Source: CAD feature listing. Evaluate the final solid. Frame: model axes, mm. A direction names the side the tool comes from. Give positions to 0.01 mm unless a question says otherwise; leave off trailing zeros. Write each loop counter-clockwise with the first axis right and the second up, starting at its lowest first coordinate (ties: lowest second). Pieces come first, ordered by that corner, then holes. Notation, with made-up numbers: (-8, 5) -> (4, 5) arc R27 cw to (4, 43) -> close; hole circle Ø1 at (72, 82). An arc over 180 degrees is marked (long way). Write item = value, one per line.
from build123d import *

# Parameters (mm, degrees)
SKETCH1_R            = 18.25
BOSS_EXTRUDE1_DEPTH  = 44.5
BOSS_EXTRUDE2_DEPTH  = 32
SKETCH3_R            = 4.75
CUT_EXTRUDE2_DEPTH   = 32
CUT_EXTRUDE3_DEPTH   = 32
SKETCH5_R            = 14.25
CUT_EXTRUDE4_DEPTH   = 4
CHAMFER1_SIZE        = 0.5
FILLET1_R            = 0.75
SKETCH6_R            = 12
CUT_EXTRUDE5_DEPTH   = 3
SKETCH7_R            = 13
BOSS_EXTRUDE3_DEPTH  = 5.5
FILLET2_R            = 1.8
SKETCH8_R            = 15.875
BOSS_EXTRUDE4_DEPTH  = 3.75
SKETCH9_R            = 14.5
BOSS_EXTRUDE5_DEPTH  = 4.75
SKETCH10_R           = 15.875
BOSS_EXTRUDE6_DEPTH  = 3.75
FILLET3_R            = 1
FILLET3_OF_MIRROR1_R = 1
SKETCH11_R           = 12.75
CUT_EXTRUDE6_DEPTH   = 79.75
SKETCH12_R           = 8
CUT_EXTRUDE7_DEPTH   = 32.75


with BuildPart() as part:
    # Sketch1 → Boss-Extrude1 (new body)
    with BuildSketch(Plane(origin=(0, 0, 0), x_dir=(1, 0, 0), z_dir=(0, 1, 0))):
        with Locations(Location((0, 0, 0), (0, 0, 270))):
            Circle(SKETCH1_R)
    extrude(amount=BOSS_EXTRUDE1_DEPTH)

    # Sketch2 → Boss-Extrude2 (add)
    with BuildSketch(Plane.XZ):
        with BuildLine():
            Line((25.5, 0), (25.5, -43))
            Line((25.5, -43), (-25.5, -43))
            Line((-25.5, -43), (-25.5, 0))
            ThreePointArc((-25.5, 0), (-20.032746784, 3.769396236), (-15.896474532, 8.964630358))
            ThreePointArc((-15.896474532, 8.964630358), (0, -18.25), (15.896474532, 8.964630358))
            ThreePointArc((15.896474532, 8.964630358), (20.032746784, 3.769396236), (25.5, 0))
        make_face()
    extrude(amount=-BOSS_EXTRUDE2_DEPTH)

    # Sketch3 → Cut-Extrude2 (cut)
    with BuildSketch(Plane(origin=(0, 32, 0), x_dir=(1, 0, 0), z_dir=(0, 1, 0))):
        with Locations(Location((-16.5, 34.25, 0), (0, 0, 270))):
            Circle(SKETCH3_R)
        with Locations(Location((16.5, 34.25, 0), (0, 0, 90))):
            Circle(SKETCH3_R)
    extrude(amount=-CUT_EXTRUDE2_DEPTH, mode=Mode.SUBTRACT)

    # Sketch4 → Cut-Extrude3 (cut)
    with BuildSketch(Plane(origin=(0, 32, 0), x_dir=(1, 0, 0), z_dir=(0, 1, 0))):
        with BuildLine():
            Line((16.25, 43), (-16.25, 43))
            ThreePointArc((-16.25, 43), (-11.008714433, 41.194952561), (-7.860592425, 36.632212324))
            ThreePointArc((-7.860592425, 36.632212324), (-5.818294481, 32.970747376), (-2.07874831, 31.075199726))
            ThreePointArc((-2.07874831, 31.075199726), (-1.040129155, 31.016729364), (0, 31))
            ThreePointArc((0, 31), (1.040129155, 31.016729364), (2.07874831, 31.075199726))
            ThreePointArc((2.07874831, 31.075199726), (5.818294481, 32.970747376), (7.860592425, 36.632212324))
            ThreePointArc((7.860592425, 36.632212324), (11.008714433, 41.194952561), (16.25, 43))
        make_face()
        with BuildLine():
            Line((-16.75, 43), (-25.5, 43))
            Line((-25.5, 43), (-25.5, 34.25))
            ThreePointArc((-25.5, 34.25), (-22.901195105, 40.401195105), (-16.75, 43))
        make_face()
        with BuildLine():
            Line((25.5, 43), (16.75, 43))
            ThreePointArc((16.75, 43), (22.901195105, 40.401195105), (25.5, 34.25))
            Line((25.5, 34.25), (25.5, 43))
        make_face()
    extrude(amount=-CUT_EXTRUDE3_DEPTH, mode=Mode.SUBTRACT)

    # Sketch5 → Cut-Extrude4 (cut)
    with BuildSketch(Plane(origin=(0, 44.5, 0), x_dir=(1, 0, 0), z_dir=(0, 1, 0))):
        with Locations(Location((0, 0, 0), (0, 0, 270))):
            Circle(SKETCH5_R)
    extrude(amount=-CUT_EXTRUDE4_DEPTH, mode=Mode.SUBTRACT)

    # Chamfer1
    chamfer1_edges = [part.edges().sort_by_distance(p)[0] for p in [
        (0, 44.5, -14.25),
    ]]
    chamfer(chamfer1_edges, length=CHAMFER1_SIZE)

    # Fillet1
    fillet1_edges = [part.edges().sort_by_distance(p)[0] for p in [
        (0, 44.5, -18.25),
    ]]
    fillet(fillet1_edges, radius=FILLET1_R)

    # Sketch6 → Cut-Extrude5 (cut)
    with BuildSketch(Plane(origin=(0, 40.5, 0), x_dir=(1, 0, 0), z_dir=(0, 1, 0))):
        with Locations(Location((0, 0, 0), (0, 0, 270))):
            Circle(SKETCH6_R)
    extrude(amount=-CUT_EXTRUDE5_DEPTH, mode=Mode.SUBTRACT)

    # Sketch7 → Boss-Extrude3 (add)
    with BuildSketch(Plane.XZ):
        with Locations(Location((0, 0, 0), (0, 0, 90))):
            Circle(SKETCH7_R)
    extrude(amount=BOSS_EXTRUDE3_DEPTH)

    # Fillet2
    fillet2_edges = [part.edges().sort_by_distance(p)[0] for p in [
        (0, -5.5, -13),
    ]]
    fillet(fillet2_edges, radius=FILLET2_R)

    # Sketch8 → Boss-Extrude4 (add)
    with BuildSketch(Plane.ZY.offset(25.5)):
        with Locations((-16.5, 16)):
            Circle(SKETCH8_R)
    boss_extrude4 = extrude(amount=BOSS_EXTRUDE4_DEPTH)

    # Sketch9 → Boss-Extrude5 (add)
    with BuildSketch(Plane.ZY.offset(29.25)):
        with Locations((-16.5, 16)):
            Circle(SKETCH9_R)
    boss_extrude5 = extrude(amount=BOSS_EXTRUDE5_DEPTH)

    # Sketch10 → Boss-Extrude6 (add)
    with BuildSketch(Plane.ZY.offset(34)):
        with Locations((-16.5, 16)):
            Circle(SKETCH10_R)
    boss_extrude6 = extrude(amount=BOSS_EXTRUDE6_DEPTH)

    # Fillet3
    fillet3_edges = [part.edges().sort_by_distance(p)[0] for p in [
        (-37.75, 16, -32.375),
    ]]
    fillet(fillet3_edges, radius=FILLET3_R)

    # Mirror1: Boss-Extrude4, Boss-Extrude5, Boss-Extrude6 across plane
    add(boss_extrude4.mirror(Plane(origin=(0, 0, 0), x_dir=(0, 0, 1), z_dir=(1, 0, 0))))
    add(boss_extrude5.mirror(Plane(origin=(0, 0, 0), x_dir=(0, 0, 1), z_dir=(1, 0, 0))))
    add(boss_extrude6.mirror(Plane(origin=(0, 0, 0), x_dir=(0, 0, 1), z_dir=(1, 0, 0))))

    # Fillet3 of Mirror1
    fillet3_of_mirror1_edges = [part.edges().sort_by_distance(p)[0] for p in [
        (37.75, 16, -32.375),
    ]]
    fillet(fillet3_of_mirror1_edges, radius=FILLET3_OF_MIRROR1_R)

    # Sketch11 → Cut-Extrude6 (cut)
    with BuildSketch(Plane.ZY.offset(37.75)):
        with Locations((-16.5, 16)):
            Circle(SKETCH11_R)
    extrude(amount=-CUT_EXTRUDE6_DEPTH, mode=Mode.SUBTRACT)

    # Sketch12 → Cut-Extrude7 (cut)
    with BuildSketch(Plane(origin=(0, 37.5, 0), x_dir=(1, 0, 0), z_dir=(0, 1, 0))):
        with Locations(Location((0, 0, 0), (0, 0, 270))):
            Circle(SKETCH12_R)
    extrude(amount=-CUT_EXTRUDE7_DEPTH, mode=Mode.SUBTRACT)


solid = part.part
(1) Material intervals for line 1 (Z direction, x = -16, y = 20); line 2 (Z direction, x = 16.5, y = 8.5); line 3 (X direction, y = 23, z = -30.5), sorted ascending.
Values follow:
line_1 = -42.99 to -38.97, -29.53 to -28.61, -4.39 to 8.79
line_2 = -43 to -39, -29.5 to -26.81, -6.19 to 7.98
line_3 = -37.38 to -34, -29.25 to -19.42, -13.58 to 13.58, 19.42 to 29.25, 34 to 37.38
(2) Access query for faces 1 (the face through (7.91, -1.824, -10.316)), 2 (the face through (-34, 3.1, -9.5)), 3 (the face through (-12, 44.5, -9)), 4 (the face through (-2, 37.5, 8)), 5 (the face through (10.95, 16.22, -41.15)). Directions: +Z, -Z, +X, -X, +Y, -Y. A direction counts if a zero-diameter tool reaches every point of the face in a straight line with its end or side. Return the directions, or none.
Values follow:
face_1 = -Y
face_2 = none
face_3 = +Z, -Z, +X, -X, +Y
face_4 = +Y
face_5 = -Z, +Y, -Y
(3) Section query A-A (y = 21). Give the number of separate pieces and of enclosed holes in the cut face, plus the area to 3 significant figures.
Values follow:
separate_pieces = 2
enclosed_holes = 2
area = 1,150 mm2
(4) First-contact query: pin 1 (4 mm diameter, centred on x = -9.5, y = 24, fed in from -Z); pin 2 (2 mm diameter, centred on y = 7.5, z = -30.5, fed in from -X); pin 3 (19 mm diameter, centred on x = 3, z = -1.5, fed in from +Y); pin 4 (7.5 mm diameter, centred on x = 16.5, z = -34.25, fed in from +Y). Flat tips, straight axial feed; report the tip coordinate or a pass-through.
Values follow:
pin_1 = -41.54
pin_2 = -37.61
pin_3 = 40.5
pin_4 = through
(5) Section query B-B (y = -2). Return loops of the section in (x, z), plus the area to 3 significant figures.
Values follow:
outline = circle Ø26 at (0, 0)
area = 531 mm2
(6) Pull-direction query (X, two-part tool) for faces 6 (the face through (27.35, 1.92, -9.17)), 7 (the face through (-3.06, 21.35, 7.39)), 8 (the face through (20, 15.8, 3.8)), 9 (the face through (-37.75, 20, -4)); classes: pulls with the +X half, pulls with the -X half, needs draft (parallel to the pull), parting line crosses it, or undercut.
Values follow:
face_6 = needs draft
face_7 = undercut
face_8 = pulls with the +X half
face_9 = pulls with the -X half
